The listing builds one solid part. Answer for the finished solid, in the listing's coordinates (mm). Coordinates: 2 decimals unless noted, no trailing zeros. Order: outer loops, then holes, each group sorted by start corner. A loop starts at its lowest first (then second) coordinate and runs counter-clockwise, first axis right, second up. Notation, with made-up numbers: (31, 14) - (37, 14) arc R18 cw to (37, 36) - close; hole circle Ø10 at (-24.5, 37). An arc over 180 degrees is marked (long way). Use a Markdown table: item, result. Add a question column.
Item 1: The part is cut by section D-D, the plane z = 20.25. Give the vertices of the cut face in (x, y), then the cut area to 3 significant figures.
Item 2: Find the intervals of material crossed by line 1 along Y through (x, z) = (0.8, 16); line 2 along Z through (x, y) = (0.55, -2) (3 decimals); line 3 along Z through (x, y) = (0.9, 3) (3 decimals), in increasing order.
Item 3: The part is cut by section A-A, the plane y = 0. Give the vertices of the cut face in (x, z) (1 decimal), then the cut area to 3 significant figures.
Item 4: The part is cut by section B-B, the plane z = 17. Give the vertices of the cut face in (x, y), then the cut area to 3 significant figures.
Item 5: The part is cut by section C-C, the plane x = 0.9. Give the vertices of the cut face in (y, z) (1 decimal), then the cut area to 3 significant figures.
from build123d import *

# Parameters (mm, degrees)
BOSS_EXTRUDE1_DEPTH     = 1.5875
F_1_4_CLEARANCE_HOLE1_D = 6.5278


with BuildPart() as part:
    # Sketch1 → Boss-Extrude1 (new body)
    with BuildSketch(Plane(origin=(0, 0, 0), x_dir=(0, 0, -1), z_dir=(1, 0, 0))):
        with BuildLine():
            Line((3.175, -7.9375), (3.175, 7.9375))
            Line((3.175, 7.9375), (-15.875, 7.9375))
            ThreePointArc((-15.875, 7.9375), (-23.8125, 0), (-15.875, -7.9375))
            Line((-15.875, -7.9375), (3.175, -7.9375))
        make_face()
    extrude(amount=BOSS_EXTRUDE1_DEPTH)

    # 1/4 Clearance Hole1 (through all)
    with Locations(Plane(origin=(1.5875, 0, 0), x_dir=(0, 0, -1), z_dir=(1, 0, 0))):
        with Locations((-15.875, 0)):
            Hole(F_1_4_CLEARANCE_HOLE1_D / 2)


solid = part.part
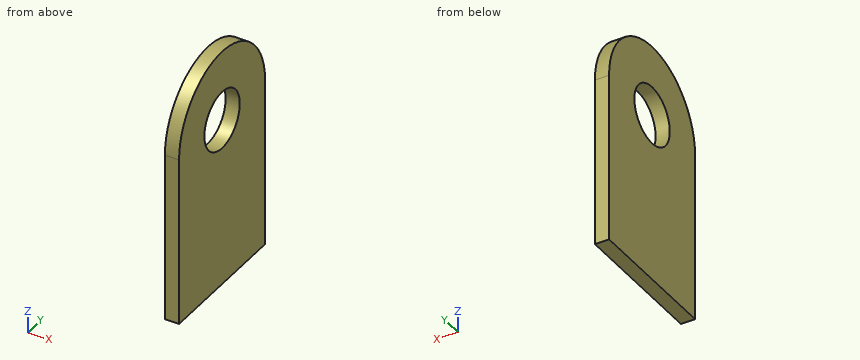
Solution:
| question | item | result |
|---|---|---|
| 1 | outline | (0, -6.62) - (1.59, -6.62) - (1.59, 6.62) - (0, 6.62) - close |
| 1 | area | 21.0 mm2 |
| 2 | line 1 | y = -7.94 to -3.26, 3.26 to 7.94 |
| 2 | line 2 | z = -3.175 to 13.296, 18.454 to 23.556 |
| 2 | line 3 | z = -3.175 to 14.589, 17.161 to 23.224 |
| 3 | outline | (0, -3.2) - (1.6, -3.2) - (1.6, 12.6) - (0, 12.6) - close; (0, 19.1) - (1.6, 19.1) - (1.6, 23.8) - (0, 23.8) - close |
| 3 | area | 32.5 mm2 |
| 4 | outline | (0, -7.86) - (1.59, -7.86) - (1.59, -3.06) - (0, -3.06) - close; (0, 3.06) - (1.59, 3.06) - (1.59, 7.86) - (0, 7.86) - close |
| 4 | area | 15.2 mm2 |
| 5 | outline | (-7.9, -3.2) - (7.9, -3.2) - (7.9, 15.9) arc R7.9 ccw to (-7.9, 15.9) - close; hole circle Ø6.5 at (0, 15.9) |
| 5 | area | 368 mm2 |
